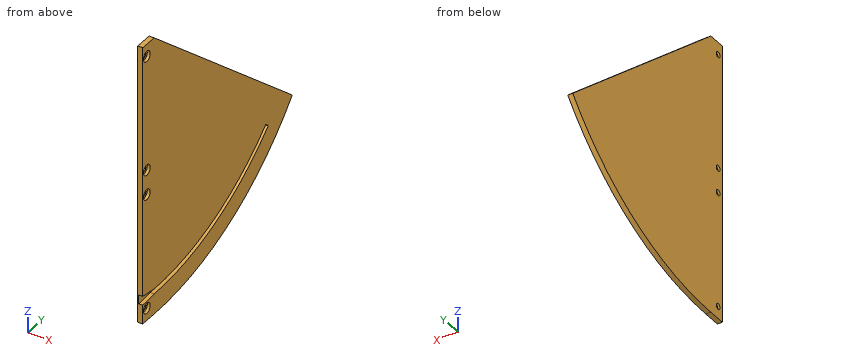
```python
from build123d import *

# Parameters (mm, degrees)
BOSS_EXTRUDE1_DEPTH = 3.175
SKETCH2_W           = 3.175
SKETCH2_H           = 178.054
BOSS_EXTRUDE2_DEPTH = 11.303
SKETCH3_R           = 1.8288
CUT_EXTRUDE1_DEPTH  = 4.175
CUT_EXTRUDE2_DEPTH  = 2.54
SKETCH8_R           = 3.3274
CUT_EXTRUDE3_DEPTH  = 1.8542


with BuildPart() as part:
    # Sketch1 → Boss-Extrude1 (new body)
    with BuildSketch(Plane(origin=(0, 0, 0), x_dir=(0, 0, -1), z_dir=(1, 0, 0))):
        with BuildLine():
            Line((0, 0), (178.054, 0))
            ThreePointArc((178.054, 0), (161.371726713, 75.248871976), (114.450905055, 136.397277275))
            Line((114.450905055, 136.397277275), (0, 0))
        make_face()
    extrude(amount=BOSS_EXTRUDE1_DEPTH)

    # Sketch2 → Boss-Extrude2 (add)
    with BuildSketch(Plane.XZ):
        with Locations((1.5875, -89.027)):
            Rectangle(SKETCH2_W, SKETCH2_H)
    extrude(amount=BOSS_EXTRUDE2_DEPTH)

    # Sketch3 → Cut-Extrude1 (cut, through all)
    with BuildSketch(Plane(origin=(3.175, 0, 0), x_dir=(0, 0, -1), z_dir=(1, 0, 0))):
        with Locations((7.874, -7.239)):
            Circle(SKETCH3_R)
        with Locations((81.153, -7.239)):
            Circle(SKETCH3_R)
        with Locations((96.901, -7.239)):
            Circle(SKETCH3_R)
        with Locations((170.18, -7.239)):
            Circle(SKETCH3_R)
    extrude(amount=-CUT_EXTRUDE1_DEPTH, mode=Mode.SUBTRACT)

    # Sketch6 → Cut-Extrude2 (cut)
    with BuildSketch(Plane(origin=(3.175, 0, 0), x_dir=(0, 0, -1), z_dir=(1, 0, 0))):
        with BuildLine():
            Line((165.1, 0), (165.982635189, -11.303))
            Line((165.982635189, -11.303), (160.260021408, -11.303))
            Line((160.260021408, -11.303), (161.925, 0))
            ThreePointArc((161.925, 0), (150.657864695, 59.345711137), (118.424448135, 110.432584453))
            Line((118.424448135, 110.432584453), (120.746496137, 112.597929246))
            ThreePointArc((120.746496137, 112.597929246), (153.611940474, 60.509352532), (165.1, 0))
        make_face()
    extrude(amount=-CUT_EXTRUDE2_DEPTH, mode=Mode.SUBTRACT)

    # Sketch8 → Cut-Extrude3 (cut)
    with BuildSketch(Plane(origin=(3.175, 0, 0), x_dir=(0, 0, -1), z_dir=(1, 0, 0))):
        with Locations((7.874, -7.239)):
            Circle(SKETCH8_R)
        with Locations((81.153, -7.239)):
            Circle(SKETCH8_R)
        with Locations((96.901, -7.239)):
            Circle(SKETCH8_R)
        with Locations((170.18, -7.239)):
            Circle(SKETCH8_R)
    extrude(amount=-CUT_EXTRUDE3_DEPTH, mode=Mode.SUBTRACT)


solid = part.part
```
Geometry: final body of the model. Coordinates: model frame, mm. Round coordinates to 2 decimals unless told otherwise and drop trailing zeros. Order: outer loops, then holes, each group sorted by start corner. A loop starts at its lowest first (then second) coordinate and runs counter-clockwise, first axis right, second up. Notation, with made-up numbers: M -33,0.5 L 22,0.5 A17 cw 22,24.5 Z; hole C -11,39.25 d4. An arc over 180 degrees is marked long. Use one line per item in the form item = value. Start each with the question number.
Q1. Cut plane A-A (x = 1.95). Count the separate pieces of the cut face and the enclosed holes in it, and give its area (3 significant figures).
Q2. Cut plane D-D (z = -32). Return loops of the section in (x, y) (3 decimals), and give its area (3 significant figures).
Q3. Cut plane C-C (y = 67). Return loops of the section in (x, z) (3 decimals), and give its area (3 significant figures).
Q4. Cut plane B-B (z = -125). Return loops of the section in (x, y) (3 decimals).
Q5. Pin query (flat end, axial travel): pin 1 Ø3.5 at (y, z) = (-6.5, -97) entering from +X. Return the tip coordinate at first contact, or that it passes through.
Q6. Material intervals for line 1 (Y direction, x = 1.95, z = -146); line 2 (Y direction, x = 2.65, z = -82); line 3 (Z direction, x = 1, y = 81.5), sorted ascending. Write a range as [from, to].
Geometry results:
q1.separate_pieces = 1
q1.enclosed_holes = 4
q1.area = 15,300 mm^2
q2.outline = M 0,-11.303 L 3.175,-11.303 L 3.175,38.136 L 0,38.136 Z
q2.area = 157 mm^2
q3.outline = M 0,-164.967 L 3.175,-164.967 L 3.175,-150.894 L 0.635,-150.894 L 0.635,-147.413 L 3.175,-147.413 L 3.175,-56.22 L 0,-56.22 Z
q3.area = 336 mm^2
q4.outline = M 0,-11.303 L 3.175,-11.303 L 3.175,102.931 L 0.635,102.931 L 0.635,107.856 L 3.175,107.856 L 3.175,126.8 L 0,126.8 Z
q5.pin_1 = 1.32
q6.line_1 = [-11.3, 70.03], [77.08, 101.92]
q6.line_2 = [-11.3, -10.46], [-4.02, 97.72]
q6.line_3 = [-158.31, -143.58], [-139.92, -68.39]
